```python
from build123d import *

# Parameters (mm, degrees)
SKETCH1_R             = 40
BOSS_EXTRUDE1_DEPTH   = 5
SKETCH2_R             = 15
SKETCH2_R_2           = 12
BOSS_EXTRUDE2_DEPTH   = 3
SKETCH3_R             = 12
CUT_EXTRUDE1_DEPTH    = 57.789083458
F_5_0MM_DOWEL_HOLE1_D = 5
CIRPATTERN1_COUNT     = 4


with BuildPart() as part:
    # Sketch1 → Boss-Extrude1 (new body)
    with BuildSketch(Plane(origin=(0, 0, 0), x_dir=(1, 0, 0), z_dir=(0, 1, 0))):
        with Locations(Location((0, 0, 0), (0, 0, 270))):
            Circle(SKETCH1_R)
    extrude(amount=BOSS_EXTRUDE1_DEPTH)

    # Sketch2 → Boss-Extrude2 (add)
    with BuildSketch(Plane(origin=(0, 5, 0), x_dir=(1, 0, 0), z_dir=(0, 1, 0))):
        with Locations(Location((0, 0, 0), (0, 0, 270))):
            Circle(SKETCH2_R)
        with Locations(Location((0, 0, 0), (0, 0, 270))):
            Circle(SKETCH2_R_2, mode=Mode.SUBTRACT)
    extrude(amount=BOSS_EXTRUDE2_DEPTH)

    # Sketch3 → Cut-Extrude1 (cut, through all)
    with BuildSketch(Plane(origin=(0, 5, 0), x_dir=(1, 0, 0), z_dir=(0, 1, 0))):
        with Locations(Location((0, 0, 0), (0, 0, 270))):
            Circle(SKETCH3_R)
    extrude(amount=-CUT_EXTRUDE1_DEPTH, mode=Mode.SUBTRACT)

    # Ø5.0mm Dowel Hole1 (through all)
    with Locations(Plane(origin=(0, 5, -27.5), x_dir=(0, 0, 1), z_dir=(0, 1, 0))):
        with Locations((0, 0)):
            f_5_0mm_dowel_hole1 = Hole(F_5_0MM_DOWEL_HOLE1_D / 2)

    # CirPattern1: Ø5.0mm Dowel Hole1 ×4 about axis
    cirpattern1_axis = Axis((0, 0, 0), (0, 1, 0))
    for i in range(1, CIRPATTERN1_COUNT):
        add(f_5_0mm_dowel_hole1.rotate(cirpattern1_axis, i * 360 / CIRPATTERN1_COUNT), mode=Mode.SUBTRACT)


solid = part.part
```
Geometry: final body of the model. Coordinates: model frame, mm. A direction names the side the tool comes from. Give positions to 0.01 mm unless a question says otherwise; leave off trailing zeros. Write each loop counter-clockwise with the first axis right and the second up, starting at its lowest first coordinate (ties: lowest second). Pieces come first, ordered by that corner, then holes.
1. Section query C-C, the plane z = 27.5. Return loops of the section in (x, y).
2. Reachability of faces 4 (the flat face through (-8.3, 0, -9.4)), 5 (the cylindrical face through (0.66, 6.479, -14.985)) from +Z, -Z, +X, -X, +Y, -Y: full face, straight path, thin tool, end or side. Return the list, or none.
3. Draft query along X for faces 1 (the flat face through (1, 5, 17)), 2 (the cylindrical face through (0, 2, -25)), 3 (the cylindrical face through (-39.05, 2.46, -8.67)). Return one class per face: released by +X, released by -X, zero draft, split by the parting line, or undercut.
4. Pin query (flat end, axial travel): P1, Ø1, axis at x = -28, y = 4, coming from the -Z side; P2, Ø6, axis at x = 27.5, z = 0, coming from the -Y side; P3, Ø2, axis at x = 10, y = 1, coming from the +Z side; P4, Ø8, axis at x = 0, z = 27.5, coming from the +Y side. Return the tip coordinate at first contact, or that it passes through.
5. Section query B-B, the plane x = 0. Return loops of the section in (y, z).
6. Section query A-A, the plane z = 0. Return loops of the section in (x, y).
7. Line query: probe 1 along Y at (x, z) = (19.5, -33); probe 2 along X at (y, z) = (3.4, 27.5); probe 3 along Z at (x, y) = (-6, 3.25). Output: solid intervals per line, ascending.
8. Section query D-D, the plane y = 1.25. Return loops of the section in (x, z).
Computed:
1. outline: (-29.05, 0) - (-2.5, 0) - (-2.5, 5) - (-29.05, 5) - close; (2.5, 0) - (29.05, 0) - (29.05, 5) - (2.5, 5) - close
2. face 4: +Z, -Z, +X, -X, -Y
2. face 5: +Y
3. face 1: zero draft
3. face 2: undercut
3. face 3: split by the parting line
4. P1: stops at z = -29.05
4. P2: stops at y = 0
4. P3: stops at z = 38.97
4. P4: stops at y = 5
5. outline: (0, -40) - (5, -40) - (5, -30) - (0, -30) - close; (0, -25) - (5, -25) - (5, -15) - (8, -15) - (8, -12) - (0, -12) - close; (0, 12) - (8, 12) - (8, 15) - (5, 15) - (5, 25) - (0, 25) - close; (0, 30) - (5, 30) - (5, 40) - (0, 40) - close
6. outline: (-40, 0) - (-30, 0) - (-30, 5) - (-40, 5) - close; (-25, 0) - (-12, 0) - (-12, 8) - (-15, 8) - (-15, 5) - (-25, 5) - close; (12, 0) - (25, 0) - (25, 5) - (15, 5) - (15, 8) - (12, 8) - close; (30, 0) - (40, 0) - (40, 5) - (30, 5) - close
7. probe 1: y = 0 to 5
7. probe 2: x = -29.05 to -2.5, 2.5 to 29.05
7. probe 3: z = -39.55 to -10.39, 10.39 to 39.55
8. outline: circle Ø80 at (0, 0); hole circle Ø5 at (-27.5, 0); hole circle Ø24 at (0, 0); hole circle Ø5 at (0, -27.5); hole circle Ø5 at (0, 27.5); hole circle Ø5 at (27.5, 0)
